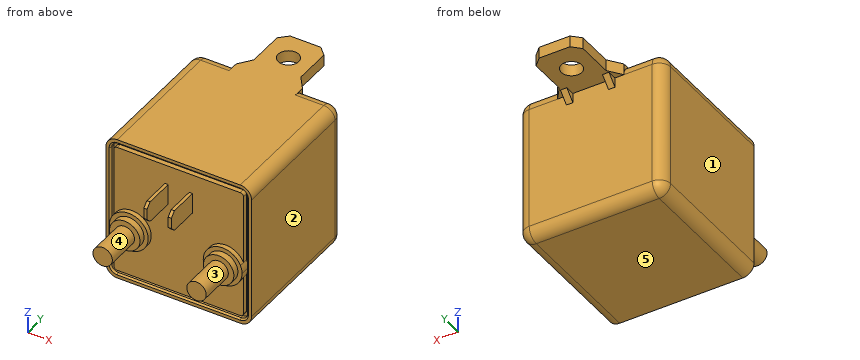
from build123d import *

# Parameters (mm, degrees)
SKETCH_1_W                 = 45
SKETCH_1_H                 = 45
EXTRUDE_1_DEPTH            = 45
FILLET_1_R                 = 3.5
EXTRUDE_2_DEPTH            = 18
EXTRUDE_2_DEPTH_BACK       = 5
SKETCH_2_W                 = 14.5
SKETCH_2_H                 = 3.5
SKETCH_4_W                 = 3
SKETCH_4_H                 = 3.5
EXTRUDE_3_DEPTH            = 3.5
CHAMFER_1_SIZE             = 2.5
SKETCH_5_R                 = 3.175
CUT_EXTRUDE_1_DEPTH        = 3.5
SKETCH_6_W                 = 2
SKETCH_6_H                 = 3
EXTRUDE_4_DEPTH            = 3
CHAMFER_2_SIZE             = 3
CHAMFER_2_OF_MIRROR_2_SIZE = 3
CUT_EXTRUDE_2_DEPTH        = 1.5
CHAMFER_3_SIZE             = 0.5
SKETCH_8_W                 = 1
SKETCH_8_H                 = 6.35
EXTRUDE_5_DEPTH            = 10.5
EXTRUDE_START              = -2
EXTRUDE_6_DEPTH            = 3.5
SKETCH_10_R                = 4.7
EXTRUDE_7_DEPTH            = 2
SKETCH_11_R                = 3
EXTRUDE_8_DEPTH            = 11
CHAMFER_4_SIZE             = 1.5


with BuildPart() as part:
    # ｽｹｯﾁ1 → ﾎﾞｽ - 押し出し1 (new body)
    with BuildSketch(Plane(origin=(0, 0, 0), x_dir=(1, 0, 0), z_dir=(0, 1, 0))):
        Rectangle(SKETCH_1_W, SKETCH_1_H)
    extrude(amount=EXTRUDE_1_DEPTH)

    # ﾌｨﾚｯﾄ1
    fillet_1_edges = [part.edges().sort_by_distance(p)[0] for p in [
        (-22.5, 45, 0),
        (0, 45, 22.5),
        (22.5, 45, 0),
        (22.5, 22.5, 22.5),
        (-22.5, 22.5, 22.5),
        (-22.5, 22.5, -22.5),
        (22.5, 22.5, -22.5),
        (0, 45, -22.5),
    ]]
    fillet(fillet_1_edges, radius=FILLET_1_R)

    # ｽｹｯﾁ2 → ﾎﾞｽ - 押し出し2 (add, two sides: drawn at the far end of the back side and taken through both)
    with BuildSketch(Plane(origin=(0, 45, 0), x_dir=(1, 0, 0), z_dir=(0, 1, 0)).offset(-EXTRUDE_2_DEPTH_BACK)):
        with Locations((0, -20.75)):
            Rectangle(SKETCH_2_W, SKETCH_2_H)
    extrude(amount=EXTRUDE_2_DEPTH + EXTRUDE_2_DEPTH_BACK)

    # ｽｹｯﾁ4 → ﾎﾞｽ - 押し出し3 (add)
    with BuildSketch(Plane.XY.offset(22.5)):
        Polygon((-7.25, 45), (-7.25, 49), (-10.25, 45), align=None)
        with Locations((-8.75, 43.25)):
            Rectangle(SKETCH_4_W, SKETCH_4_H)
    extrude_3 = extrude(amount=-EXTRUDE_3_DEPTH)

    # ﾐﾗｰ1: ﾎﾞｽ - 押し出し3 across plane
    add(extrude_3.mirror(Plane(origin=(0, 0, 0), x_dir=(0, 0, 1), z_dir=(1, 0, 0))))

    # 面取り1
    chamfer_1_edges = [part.edges().sort_by_distance(p)[0] for p in [
        (-7.25, 63, 20.75),
        (7.25, 63, 20.75),
    ]]
    chamfer(chamfer_1_edges, length=CHAMFER_1_SIZE)

    # ｽｹｯﾁ5 → ｶｯﾄ - 押し出し1 (cut)
    with BuildSketch(Plane(origin=(0, 0, 19), x_dir=(-1, 0, 0), z_dir=(0, 0, -1))):
        with Locations((0, 54.525)):
            Circle(SKETCH_5_R)
    extrude(amount=-CUT_EXTRUDE_1_DEPTH, mode=Mode.SUBTRACT)

    # ｽｹｯﾁ6 → ﾎﾞｽ - 押し出し4 (add)
    with BuildSketch(Plane(origin=(0, 0, 19), x_dir=(-1, 0, 0), z_dir=(0, 0, -1))):
        with Locations((-6.5, 46.5)):
            Rectangle(SKETCH_6_W, SKETCH_6_H)
    extrude_4 = extrude(amount=EXTRUDE_4_DEPTH)

    # 面取り2
    chamfer_2_edges = [part.edges().sort_by_distance(p)[0] for p in [
        (6.5, 48, 16),
    ]]
    chamfer(chamfer_2_edges, length=CHAMFER_2_SIZE - 0.0001)  # a hair under: the kernel refuses the full size

    # ﾐﾗｰ2: ﾎﾞｽ - 押し出し4 across plane
    add(extrude_4.mirror(Plane(origin=(0, 0, 0), x_dir=(0, 0, 1), z_dir=(1, 0, 0))))

    # 面取り2 of ﾐﾗｰ2
    chamfer_2_of_mirror_2_edges = [part.edges().sort_by_distance(p)[0] for p in [
        (-6.5, 48, 16),
    ]]
    chamfer(chamfer_2_of_mirror_2_edges, length=CHAMFER_2_OF_MIRROR_2_SIZE - 0.0001)  # a hair under: the kernel refuses the full size

    # ｽｹｯﾁ7 → ｶｯﾄ - 押し出し2 (cut)
    with BuildSketch(Plane.XZ):
        with BuildLine():
            Line((21, -19), (21, 19))
            ThreePointArc((21, 19), (20.414213562, 20.414213562), (19, 21))
            Line((19, 21), (-19, 21))
            ThreePointArc((-19, 21), (-20.414213562, 20.414213562), (-21, 19))
            Line((-21, 19), (-21, -19))
            ThreePointArc((-21, -19), (-20.414213562, -20.414213562), (-19, -21))
            Line((-19, -21), (19, -21))
            ThreePointArc((19, -21), (20.414213562, -20.414213562), (21, -19))
        make_face()
        with BuildLine():
            ThreePointArc((20, 19), (19.707106781, 19.707106781), (19, 20))
            Line((19, 20), (-19, 20))
            ThreePointArc((-19, 20), (-19.707106781, 19.707106781), (-20, 19))
            Line((-20, 19), (-20, -19))
            ThreePointArc((-20, -19), (-19.707106781, -19.707106781), (-19, -20))
            Line((-19, -20), (19, -20))
            ThreePointArc((19, -20), (19.707106781, -19.707106781), (20, -19))
            Line((20, -19), (20, 19))
        make_face(mode=Mode.SUBTRACT)
    extrude(amount=-CUT_EXTRUDE_2_DEPTH, mode=Mode.SUBTRACT)

    # 面取り3
    chamfer_3_edges = [part.edges().sort_by_distance(p)[0] for p in [
        (21, 0, 0),
        (20.414213562, 0, 20.414213562),
        (0, 0, 21),
        (-20.414213562, 0, 20.414213562),
        (-21, 0, 0),
        (-20.414213562, 0, -20.414213562),
        (0, 0, -21),
        (20.414213562, 0, -20.414213562),
    ]]
    chamfer(chamfer_3_edges, length=CHAMFER_3_SIZE)

    # ｽｹｯﾁ8 → ﾎﾞｽ - 押し出し5 (add)
    with BuildSketch(Plane.XZ):
        with Locations((3.75, 10.825)):
            Rectangle(SKETCH_8_W, SKETCH_8_H)
    extrude_5 = extrude(amount=EXTRUDE_5_DEPTH)

    # ｽｹｯﾁ9 → ﾎﾞｽ - 押し出し6 (add)
    with BuildSketch(Plane.XZ.offset(EXTRUDE_START)):
        with BuildLine():
            ThreePointArc((20, -7.172915762), (20.373670062, -5.999744871), (20.5, -4.775))
            ThreePointArc((20.5, -4.775), (20.373670062, -3.550255129), (20, -2.377084238))
            Line((20, -2.377084238), (20, -7.172915762))
        make_face()
        with BuildLine():
            Line((20, -7.172915762), (20, -2.377084238))
            ThreePointArc((20, -2.377084238), (8.5, -4.775), (20, -7.172915762))
        make_face()
    extrude_6 = extrude(amount=EXTRUDE_6_DEPTH)

    # ｽｹｯﾁ10 → ﾎﾞｽ - 押し出し7 (add)
    with BuildSketch(Plane.XZ.offset(1.5)):
        with Locations(Location((14.5, -4.775, 0), (0, 0, 270))):
            Circle(SKETCH_10_R)
    extrude_7 = extrude(amount=EXTRUDE_7_DEPTH)

    # ｽｹｯﾁ11 → ﾎﾞｽ - 押し出し8 (add)
    with BuildSketch(Plane.XZ.offset(3.5)):
        with Locations(Location((14.5, -4.775, 0), (0, 0, 270))):
            Circle(SKETCH_11_R)
    extrude_8 = extrude(amount=EXTRUDE_8_DEPTH)

    # ﾐﾗｰ3: ﾎﾞｽ - 押し出し5, ﾎﾞｽ - 押し出し6, ﾎﾞｽ - 押し出し7, ﾎﾞｽ - 押し出し8 across plane
    add(extrude_5.mirror(Plane(origin=(0, 0, 0), x_dir=(0, 0, 1), z_dir=(1, 0, 0))))
    add(extrude_6.mirror(Plane(origin=(0, 0, 0), x_dir=(0, 0, 1), z_dir=(1, 0, 0))))
    add(extrude_7.mirror(Plane(origin=(0, 0, 0), x_dir=(0, 0, 1), z_dir=(1, 0, 0))))
    add(extrude_8.mirror(Plane(origin=(0, 0, 0), x_dir=(0, 0, 1), z_dir=(1, 0, 0))))

    # 面取り4
    chamfer_4_edges = [part.edges().sort_by_distance(p)[0] for p in [
        (3.75, -10.5, 14),
        (3.75, -10.5, 7.65),
        (-3.75, -10.5, 7.65),
        (-3.75, -10.5, 14),
    ]]
    chamfer(chamfer_4_edges, length=CHAMFER_4_SIZE)


solid = part.part
Here's how the part is built. I have some questions about the finished solid (model axes, mm). Face numbers are marked on the shaded views. A direction names the side the tool comes from. Coordinates: 2 decimals unless noted, no trailing zeros. Order: outer loops, then holes, each group sorted by start corner. A loop starts at its lowest first (then second) coordinate and runs counter-clockwise, first axis right, second up. Notation, with made-up numbers: (18, 57.5) -> (66, 57.5) arc R22 ccw to (66, 72.5) -> close; hole circle Ø11 at (38.25, -16.5). An arc over 180 degrees is marked (long way). Answer in a Markdown table with one row per item.
(1) Please list where these lines run through material, in increasing order: probe 1 along Y at (x, z) = (0, 20.8); probe 2 along Y at (x, z) = (0, 21.8); probe 3 along Y at (x, z) = (-11, 8).
Answer key:
| item | result |
|---|---|
| probe 1 | 1.5 to 51.35, 57.7 to 63 |
| probe 2 | 0 to 51.35, 57.7 to 63 |
| probe 3 | 0 to 45 |
(2) Will these pins go through, and if not, where does the flat tip stop? pin 1 Ø1 at (x, z) = (-11, 13.5) entering from +Y; pin 2 Ø1.8 at (y, z) = (43.5, 21.5) entering from -X; pin 3 Ø1 at (y, z) = (52.5, 20.5) entering from +X.
Answer key:
| item | result |
|---|---|
| pin 1 | y = 45 |
| pin 2 | x = -21.64 |
| pin 3 | x = 7.25 |
(3) On a 3-axis mill with a long thin cutter (end or side, diameter ignored), from which of +Z, -Z, +X, -X, +Y, -Y can I reach the whole of each face in a straight line? I mean the marked faces 4 and 5. Say none if no direction works.
Answer key:
| item | result |
|---|---|
| face 4 | -Y |
| face 5 | -Z, +X, -X, +Y, -Y |
(4) Thinking about a two-plate mould opening in X: for the marked faces 1, 2 and 3, which applies, +X half, -X half, draft (parallel to the pull), parting line (faces both ways), or undercut?
Answer key:
| item | result |
|---|---|
| face 1 | -X half |
| face 2 | +X half |
| face 3 | undercut |
(5) I want a section at C-C on y = 50.5. List the corners of the cut face in (x, z) for me.
Answer key:
| item | result |
|---|---|
| outline | (-7.25, 19) -> (7.25, 19) -> (7.25, 22.5) -> (-7.25, 22.5) -> close |
(6) I want a section at D-D on x = -12.5. List the corners of the cut face in (y, z) for me, then the cut area to 3 significant figures.
Answer key:
| item | result |
|---|---|
| outline | (-14.5, -7.01) -> (-3.5, -7.01) -> (-3.5, -9.03) -> (-1.5, -9.03) -> (-1.5, -10.43) -> (0, -10.43) -> (0, -20) -> (1.5, -20) -> (1.5, -21) -> (0.5, -21) -> (0, -21.5) -> (0, -22.5) -> (41.5, -22.5) arc R3.5 ccw to (45, -19) -> (45, 19) arc R3.5 ccw to (41.5, 22.5) -> (0, 22.5) -> (0, 21.5) -> (0.5, 21) -> (1.5, 21) -> (1.5, 20) -> (0, 20) -> (0, 0.88) -> (-1.5, 0.88) -> (-1.5, -0.52) -> (-3.5, -0.52) -> (-3.5, -2.54) -> (-14.5, -2.54) -> close |
| area | 2,100 mm^2 |
(7) I want a section at A-A on x = 0. List the corners of the cut face in (y, z) for me, then the cut area to 3 significant figures.
Answer key:
| item | result |
|---|---|
| outline | (0, -22.5) -> (41.5, -22.5) arc R3.5 ccw to (45, -19) -> (45, 19) -> (51.35, 19) -> (51.35, 22.5) -> (0, 22.5) -> (0, 21.5) -> (0.5, 21) -> (1.5, 21) -> (1.5, 20) -> (0, 20) -> (0, -20) -> (1.5, -20) -> (1.5, -21) -> (0.5, -21) -> (0, -21.5) -> close; (57.7, 19) -> (63, 19) -> (63, 22.5) -> (57.7, 22.5) -> close |
| area | 2,060 mm^2 |
(8) I want a section at B-B on x = 14.5. List the corners of the cut face in (y, z) for me (3 decimals), then the cut area to 3 significant figures.
Answer key:
| item | result |
|---|---|
| outline | (-14.5, -7.775) -> (-3.5, -7.775) -> (-3.5, -9.475) -> (-1.5, -9.475) -> (-1.5, -10.775) -> (0, -10.775) -> (0, -20) -> (1.5, -20) -> (1.5, -21) -> (0.5, -21) -> (0, -21.5) -> (0, -22.5) -> (41.5, -22.5) arc R3.5 ccw to (45, -19) -> (45, 19) arc R3.5 ccw to (41.5, 22.5) -> (0, 22.5) -> (0, 21.5) -> (0.5, 21) -> (1.5, 21) -> (1.5, 20) -> (0, 20) -> (0, 1.225) -> (-1.5, 1.225) -> (-1.5, -0.075) -> (-3.5, -0.075) -> (-3.5, -1.775) -> (-14.5, -1.775) -> close |
| area | 2,120 mm^2 |
